Input: part model. Units: mm. Frame: model coordinates. A direction names the side the tool comes from. Give positions to 0.01 mm unless a question says otherwise; leave off trailing zeros. Loops run counter-clockwise (first coordinate to the right, second up) from the corner with the lowest first, then second, coordinate; pieces in that order, holes last. Notation, with made-up numbers: (21, 60.25) - (37, 60.25) arc R24 cw to (37, 77.25) - close; hole circle Ø7 at (-19, 74.5). An arc over 180 degrees is marked (long way). Answer as a JSON object with one key per item and string values. Group by question number.
(1) Section query B-B (z = -133). Return loops of the section in (x, y), plus the area to 3 significant figures.
(2) Section query A-A (y = -244). Return loops of the section in (x, z).
(3) Access query for faces 4 (the cylindrical face through (3.944, -308.494, -166.785)), 5 (the flat face through (574.8, -123, -173)). Directions: +Z, -Z, +X, -X, +Y, -Y. A direction counts if a zero-diameter tool reaches every point of the face in a straight line with its end or side. Return the directions, or none.
(4) Pin query (flat end, axial travel): P1, Ø8, axis at x = 364.5, z = -244, coming from the -Y side. Return the tip coordinate at first contact, or that it passes through.
(5) Section query D-D (y = -175.5). Return loops of the section in (x, z), plus the area to 3 significant figures.
(6) Section query C-C (z = -279.5). Return loops of the section in (x, y).
(7) Mould query, pull axis Y, two halves, no side actions, for faces 1 (the cylindrical face through (578.9, -262.1, -107.3)), 2 (the cylindrical face through (578.856, -308.494, -174.285)), 3 (the flat face through (8, -123, -168)). Classes: +Y half, -Y half, draft (parallel to the pull), parting line (faces both ways), or undercut.
(8) Material intervals for L1, parallel to X at y = -211, z = -284.5; L2, parallel to Z at x = 410, y = -5; L3, parallel to X at y = -1.25, z = -30.31, sorted ascending.
```python
from build123d import *

# Parameters (mm, degrees)
SKETCH2_W                      = 582.8
SKETCH2_H                      = 341.07
BASE_FLANGE5_DEPTH             = 8
EDGE_FLANGE2_STRIP_W           = 33.4732
EDGE_FLANGE2_STRIP_H           = 8
EDGE_FLANGE2_STRIP_CUT_DEPTH   = 341.07
EDGE_FLANGE2_STRIP_2_W         = 33.4732
EDGE_FLANGE2_STRIP_2_H         = 8
EDGE_FLANGE2_STRIP_CUT_2_DEPTH = 341.07
EDGE_FLANGE2_DEPTH             = 341.07
EDGE_FLANGE2_BEND_DEPTH        = 341.07
BOSS_EXTRUDE4_DEPTH            = 4
F_10_0MM_DOWEL_HOLE1_D         = 10
BOSS_EXTRUDE5_DEPTH            = 4
CUT_EXTRUDE2_DEPTH             = 743.413921694
CUT_EXTRUDE2_DEPTH_BACK        = 743.413921694
SKETCH40_R                     = 75
F_10_0MM_DOWEL_HOLE2_D         = 10
F_10_0MM_DOWEL_HOLE3_D         = 10


# Sheet-metal steps are written as plain solids
with BuildPart() as part:
    # Sketch2 → Base-Flange5 (new body)
    with BuildSketch(Plane(origin=(0, 0, 0), x_dir=(1, 0, 0), z_dir=(0, 1, 0))):
        with Locations((291.4, 170.535)):
            Rectangle(SKETCH2_W, SKETCH2_H)
    extrude(amount=-BASE_FLANGE5_DEPTH)

    # Edge-Flange2 strip (across the edge) → Edge-Flange2 strip cut (cut)
    with BuildSketch(Plane(origin=(0, -8, 0), x_dir=(1, 0, 0), z_dir=(0, 0, -1))):
        with Locations((-8, -4)):
            Rectangle(EDGE_FLANGE2_STRIP_W, EDGE_FLANGE2_STRIP_H)
    extrude(amount=EDGE_FLANGE2_STRIP_CUT_DEPTH, mode=Mode.SUBTRACT)

    # Edge-Flange2 strip 2 (across the edge) → Edge-Flange2 strip cut 2 (cut)
    with BuildSketch(Plane(origin=(582.8, -8, -341.07), x_dir=(-1, 0, 0), z_dir=(0, 0, 1))):
        with Locations((-8, -4)):
            Rectangle(EDGE_FLANGE2_STRIP_2_W, EDGE_FLANGE2_STRIP_2_H)
    extrude(amount=EDGE_FLANGE2_STRIP_CUT_2_DEPTH, mode=Mode.SUBTRACT)

    # Edge-Flange2 section (across the edge) → Edge-Flange2 (add)
    with BuildSketch(Plane(origin=(0, -8, 0), x_dir=(1, 0, 0), z_dir=(0, 0, -1))):
        with BuildLine():
            Line((0, 0.7366), (0, 130))
            Line((0, 130), (8, 130))
            Line((8, 130), (8, 0.7366))
            ThreePointArc((8, 0.7366), (8.215745145, 0.215745145), (8.7366, 0))
            Line((8.7366, 0), (8.7366, -8))
            ThreePointArc((8.7366, -8), (2.558890895, -5.441109105), (0, 0.7366))
        make_face()
    extrude(amount=EDGE_FLANGE2_DEPTH)

    # Edge-Flange2 section 2 (across the edge) → Edge-Flange2 bend (add)
    with BuildSketch(Plane(origin=(582.8, -8, -341.07), x_dir=(-1, 0, 0), z_dir=(0, 0, 1))):
        with BuildLine():
            Line((0, 0.7366), (0, 130))
            Line((0, 130), (8, 130))
            Line((8, 130), (8, 0.7366))
            ThreePointArc((8, 0.7366), (8.215745145, 0.215745145), (8.7366, 0))
            Line((8.7366, 0), (8.7366, -8))
            ThreePointArc((8.7366, -8), (2.558890895, -5.441109105), (0, 0.7366))
        make_face()
    extrude(amount=EDGE_FLANGE2_BEND_DEPTH)

    # Sketch39 → Boss-Extrude4 (add, symmetric)
    with BuildSketch(Plane.ZY.offset(-4)):
        with BuildLine():
            Line((-341.07, -138), (0, -138))
            ThreePointArc((0, -138), (-170.535, -308.535), (-341.07, -138))
        make_face()
    extrude(amount=BOSS_EXTRUDE4_DEPTH, both=True)

    # Ø10.0mm Dowel Hole1 (through all)
    with Locations(Plane(origin=(306.4, 0, -30.31), x_dir=(0, 0, 1), z_dir=(0, 1, 0))):
        with Locations((0, 0), (0, -30)):
            Hole(F_10_0MM_DOWEL_HOLE1_D / 2)

    # Sketch46 → Boss-Extrude5 (add, symmetric)
    with BuildSketch(Plane(origin=(578.8, 0, 0), x_dir=(0, 0, -1), z_dir=(1, 0, 0))):
        with BuildLine():
            Line((0, -138), (341.07, -138))
            ThreePointArc((341.07, -138), (170.535, -308.535), (0, -138))
        make_face()
    extrude(amount=BOSS_EXTRUDE5_DEPTH, both=True)

    # Sketch40 → Cut-Extrude2 (cut, two sides: drawn at the far end of the back side and taken through both)
    with BuildSketch(Plane.ZY.offset(-CUT_EXTRUDE2_DEPTH_BACK)):
        with Locations(Location((-170.535, -221.773804428, 0), (0, 0, 270))):
            Circle(SKETCH40_R)
    extrude(amount=CUT_EXTRUDE2_DEPTH + CUT_EXTRUDE2_DEPTH_BACK, mode=Mode.SUBTRACT)

    # Ø10.0mm Dowel Hole2 (through all)
    with Locations(Plane(origin=(372.86, 0, -46.56), x_dir=(0, 0, 1), z_dir=(0, 1, 0))):
        with Locations((0, 0), (0, 38.08)):
            Hole(F_10_0MM_DOWEL_HOLE2_D / 2)

    # Ø10.0mm Dowel Hole3 (through all)
    with Locations(Plane(origin=(410.94, 0, -208.49), x_dir=(0, 0, 1), z_dir=(0, 1, 0))):
        with Locations((0, 0), (0, -38.08)):
            Hole(F_10_0MM_DOWEL_HOLE3_D / 2)


solid = part.part
```
Recorded:
{
 "1": {"outline": "(0, -304.35) - (8, -304.35) - (8, -286.71) - (0, -286.71) - close; (0, -156.84) - (8, -156.84) - (8, -8.74) arc R0.74 cw to (8.74, -8) - (574.06, -8) arc R0.74 cw to (574.8, -8.74) - (574.8, -156.84) - (582.8, -156.84) - (582.8, -8.74) arc R8.74 ccw to (574.06, 0) - (8.74, 0) arc R8.74 ccw to (0, -8.74) - close; (574.8, -304.35) - (582.8, -304.35) - (582.8, -286.71) - (574.8, -286.71) - close", "area": "7,290 mm^2"},
 "2": {"outline": "(0, -304.12) - (8, -304.12) - (8, -242.17) - (0, -242.17) - close; (0, -98.9) - (8, -98.9) - (8, -36.95) - (0, -36.95) - close; (574.8, -304.12) - (582.8, -304.12) - (582.8, -242.17) - (574.8, -242.17) - close; (574.8, -98.9) - (582.8, -98.9) - (582.8, -36.95) - (574.8, -36.95) - close"},
 "3": {"face 4": "+X, -X, -Y", "face 5": "+Z, -Z, -Y"},
 "4": {"P1": "stops at y = -8"},
 "5": {"outline": "(0, -336.9) - (8, -336.9) - (8, -229.56) - (0, -229.56) - close; (0, -111.51) - (8, -111.51) - (8, -4.17) - (0, -4.17) - close; (574.8, -336.9) - (582.8, -336.9) - (582.8, -229.56) - (574.8, -229.56) - close; (574.8, -111.51) - (582.8, -111.51) - (582.8, -4.17) - (574.8, -4.17) - close", "area": "3,430 mm^2"},
 "6": {"outline": "(0, -269.18) - (8, -269.18) - (8, -8.74) arc R0.74 cw to (8.74, -8) - (574.06, -8) arc R0.74 cw to (574.8, -8.74) - (574.8, -269.18) - (582.8, -269.18) - (582.8, -8.74) arc R8.74 ccw to (574.06, 0) - (8.74, 0) arc R8.74 ccw to (0, -8.74) - close"},
 "7": {"face 1": "undercut", "face 2": "-Y half", "face 3": "draft"},
 "8": {"L1": "x = 0 to 8, 574.8 to 582.8", "L2": "z = -341.07 to -213.4, -203.58 to -51.47, -41.65 to 0", "L3": "x = 4.23 to 271.4, 281.4 to 301.4, 311.4 to 578.57"}
}
